from build123d import *

# Parameters (mm, degrees)
SKETCH_1_W               = 38.9
SKETCH_1_H               = 40
EXTRUDE_1_DEPTH          = 7.5
EXTRUDE_2_DEPTH          = 33.7
SKETCH_4_W               = 23.3
SKETCH_4_H               = 35.5
CUT_EXTRUDE_1_DEPTH      = 21
CUT_EXTRUDE_1_DEPTH_BACK = 21
CHAMFER_1_SIZE           = 2
HOLE_WIZARD_M81_D        = 6.8
HOLE_WIZARD_M81_DEPTH    = 5.2


with BuildPart() as part:
    # Эскиз1 → Бобышка-Вытянуть1 (new body)
    with BuildSketch(Plane(origin=(0, 0, 0), x_dir=(1, 0, 0), z_dir=(0, 1, 0))):
        Rectangle(SKETCH_1_W, SKETCH_1_H)
    extrude(amount=EXTRUDE_1_DEPTH)

    # Эскиз2 → Вырез-Повернуть1 (revolve, cut)
    with BuildSketch(Plane.XY):
        Polygon((-4, 0), (-4, 3.75), (-6.5, 3.75), (-6.5, 7.5), (0, 7.5), (0, 0), align=None)
    revolve(axis=Axis((0, 7.5, 0), (0, -1, 0)), mode=Mode.SUBTRACT)

    # Эскиз3 → Бобышка-Вытянуть2 (add)
    with BuildSketch(Plane(origin=(19.45, 0, 0), x_dir=(0, 0, -1), z_dir=(1, 0, 0))):
        with BuildLine():
            Line((-20, 7.5), (-17.35257463, 27.766749589))
            ThreePointArc((-17.35257463, 27.766749589), (0, 43), (17.35257463, 27.766749589))
            Line((17.35257463, 27.766749589), (20, 7.5))
            Line((20, 7.5), (-20, 7.5))
        make_face()
    extrude(amount=-EXTRUDE_2_DEPTH)

    # Эскиз4 → Вырез-Вытянуть1 (cut, two sides)
    with BuildSketch(Plane.XY) as cut_extrude_1_sk:
        with Locations((2.6, 25.25)):
            Rectangle(SKETCH_4_W, SKETCH_4_H)
    extrude(amount=CUT_EXTRUDE_1_DEPTH, mode=Mode.SUBTRACT)
    extrude(cut_extrude_1_sk.sketch, amount=-CUT_EXTRUDE_1_DEPTH_BACK, mode=Mode.SUBTRACT)

    # Фаска1
    chamfer_1_edges = [part.edges().sort_by_distance(p)[0] for p in [
        (-19.45, 3.75, -20),
        (-19.45, 3.75, 20),
    ]]
    chamfer(chamfer_1_edges, length=CHAMFER_1_SIZE)

    # Эскиз10 → Зенковка для винта с полупотайной головкой 1 (revolve, cut)
    with BuildSketch(Plane(origin=(19.45, 25.5, 0), x_dir=(0, 0, -1), z_dir=(0, 1, 0))):
        Polygon((0, 0), (0, 5.2), (4.25, 5.2), (4.25, 4.25), (8.5, 0), align=None)
    revolve(axis=Axis((25.8, 25.5, 0), (-1, 0, 0)), mode=Mode.SUBTRACT)

    # Отверстие обработанное метчиком M81
    with Locations(Plane.ZY.offset(14.25)):
        with Locations((0, 25.5)):
            Hole(HOLE_WIZARD_M81_D / 2, depth=HOLE_WIZARD_M81_DEPTH)


solid = part.part
Design review of the part built by this model. Coordinates are the model's own, in mm. A direction names the side the tool comes from. Coordinates: 2 decimals unless noted, no trailing zeros. Write each loop counter-clockwise with the first axis right and the second up, starting at its lowest first coordinate (ties: lowest second). Pieces come first, ordered by that corner, then holes. Notation, with made-up numbers: (9, -9) - (42, -9) arc R27 ccw to (42, 26) - close; hole circle Ø11 at (62, 16.25). An arc over 180 degrees is marked (long way). Use one line per item in the form item = value.
Q1. Machinability: for faces 4 (the flat face through (8, 7.5, 0)), 5 (the flat face through (3, 3.75, -3)), 6 (the cylindrical face through (14.73, 29.65, 0.92)), which of the approach directions +Z, -Z, +X, -X, +Y, -Y give a long, thin tool a straight path to every point of the face, cutting with its end or side? Answer none if there is none.
Taken from the geometry:
face_4 = +Z, -Z, +Y
face_5 = +Y
face_6 = +X
Q2. Insertion check: pin 1 Ø6.5 at (x, z) = (0, 0) entering from -Y; pin 2 Ø10.5 at (y, z) = (23, 0.5) entering from -X; pin 3 Ø6.5 at (x, z) = (-2.5, 2) entering from +Y; pin 4 Ø1.6 at (x, z) = (-15.5, 8) entering from +Y. Each pin has a flat end and moves straight along its axis. Give the tip position at first contact, or say it passes through.
Taken from the geometry:
pin_1 = through
pin_2 = -14.25
pin_3 = 3.75
pin_4 = 7.5
Q3. Consider section A-A (z = 0). Write out the cut boundary in (x, y), plus the area to 3 significant figures.
Taken from the geometry:
outline = (-19.45, 0) - (-4, 0) - (-4, 3.75) - (-6.5, 3.75) - (-6.5, 7.5) - (-9.05, 7.5) - (-9.05, 22.1) - (-14.25, 22.1) - (-14.25, 7.5) - (-19.45, 7.5) - close; (-14.25, 28.9) - (-9.05, 28.9) - (-9.05, 43) - (-14.25, 43) - close; (4, 0) - (19.45, 0) - (19.45, 17) - (15.2, 21.25) - (14.25, 21.25) - (14.25, 7.5) - (6.5, 7.5) - (6.5, 3.75) - (4, 3.75) - close; (14.25, 29.75) - (15.2, 29.75) - (19.45, 34) - (19.45, 43) - (14.25, 43) - close
area = 485 mm^2
Q4. The part is to be moulded in two halves that separate along Y. For faces 1 (the conical face through (15.47, 24.14, -4.31)), 2 (the flat face through (-5, 0, 0)), 3 (the flat face through (-17, 7.5, 0)), say which applies: +Y half, -Y half, draft (parallel to the pull), parting line (faces both ways), or undercut.
Taken from the geometry:
face_1 = undercut
face_2 = -Y half
face_3 = +Y half
Q5. Consider section B-B (x = 0). Write out the cut boundary in (y, z).
Taken from the geometry:
outline = (0, -20) - (7.5, -20) - (7.5, -6.5) - (3.75, -6.5) - (3.75, -4) - (0, -4) - close; (0, 4) - (3.75, 4) - (3.75, 6.5) - (7.5, 6.5) - (7.5, 20) - (0, 20) - close
Q6. Consider section C-C (y = 11.5). Write out the cut boundary in (x, z).
Taken from the geometry:
outline = (-14.25, -19.48) - (-9.05, -19.48) - (-9.05, 19.48) - (-14.25, 19.48) - close; (14.25, -19.48) - (19.45, -19.48) - (19.45, 19.48) - (14.25, 19.48) - close
Q7. For probe 1 along X at (y, z) = (2.35, 0); probe 2 along Z at (x, y) = (0, 1); probe 3 along Y at (x, z) = (-11.25, 0), list the stretches that pass through material, from the lowest coordinate up.
Taken from the geometry:
probe_1 = -19.45 to -4, 4 to 19.45
probe_2 = -20 to -4, 4 to 20
probe_3 = 0 to 22.1, 28.9 to 43
Q8. Consider section D-D (x = -11.5). Write out the cut boundary in (y, z), plus the area to 3 significant figures.
Taken from the geometry:
outline = (0, -20) - (7.5, -20) - (27.77, -17.35) arc R17.5 ccw to (27.77, 17.35) - (7.5, 20) - (0, 20) - close; hole circle Ø6.8 at (25.5, 0)
area = 1,420 mm^2
